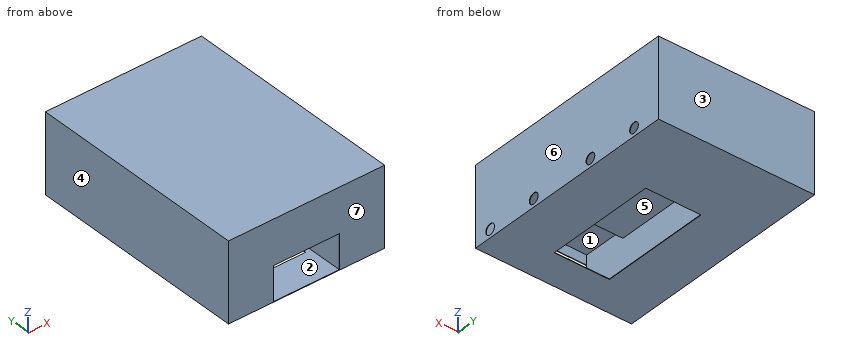
from build123d import *

# Parameters (mm, degrees)
F0_W      = 297
F0_H      = 420
F1_DEPTH  = 150
F3_START  = -1
F2_W      = 295
F2_H      = 418
F3_DEPTH  = 148
F4_W      = 125
F4_H      = 65
F5_DEPTH  = 25
F6_W      = 105
F6_H      = 210
F7_DEPTH  = 25
F9_DEPTH  = 67.5
F11_DEPTH = 295
F12_W     = 83
F12_H     = 1
F13_DEPTH = 148.5
F15_W     = 83
F15_H     = 15.0031849133
F16_DEPTH = 295
F14_W     = 83
F14_H     = 20
F17_DEPTH = 62.5
F18_R     = 10
F19_DEPTH = 7.5


with BuildPart() as f1:
    # F0 (on Top) → F1 (new body)
    with BuildSketch(Plane.XY):
        Rectangle(F0_W, F0_H)
    extrude(amount=F1_DEPTH)

    # F2 (on face) → F3 (cut)
    with BuildSketch(Plane.XY.offset(150).offset(F3_START)):
        Rectangle(F2_W, F2_H)
    extrude(amount=-F3_DEPTH, mode=Mode.SUBTRACT)

    # F4 (on face) → F5 (cut)
    with BuildSketch(Plane.XZ.offset(210)):
        with Locations((0, 33.5)):
            Rectangle(F4_W, F4_H)
    extrude(amount=-F5_DEPTH, mode=Mode.SUBTRACT)

    # F6 (on Top) → F7 (cut)
    with BuildSketch(Plane.XY):
        with Locations((0, -40)):
            Rectangle(F6_W, F6_H)
    extrude(amount=F7_DEPTH, mode=Mode.SUBTRACT)

    # F8 (on face) → F9 (join)
    with BuildSketch(Plane.XY.offset(1)):
        Polygon((-63.5, -209), (-62.5, -209), (-62.5, 65), (61.5036363636, 65), (62.5, -209), (63.5, -209), (62.5, 66), (-63.5, 66), align=None)
    extrude(amount=F9_DEPTH)

    # F10 (on face) → F11 (join, through all)
    with BuildSketch(Plane.YZ.offset(-147.5)):
        Polygon((-126, 68.5), (66, 68.5), (66, 69.5), (-125, 69.5), (-125, 85.5), (-209, 85.5), (-209.0797476204, 84.5031849133), (-126, 84.5031849133), align=None)
    extrude(amount=F11_DEPTH)

    # F12 (on Right) → F13 (join, symmetric)
    with BuildSketch(Plane.YZ):
        with Locations((-167.5, 69)):
            Rectangle(F12_W, F12_H)
    extrude(amount=F13_DEPTH, both=True)

    # F15 (on face) → F16 (join, through all)
    with BuildSketch(Plane.YZ.offset(-147.5)):
        with Locations((-167.5, 77.0015924567)):
            Rectangle(F15_W, F15_H)
    extrude(amount=F16_DEPTH)

    # F14 (on Right) → F17 (cut, symmetric)
    with BuildSketch(Plane.YZ):
        with Locations((-167.5, 74.5)):
            Rectangle(F14_W, F14_H)
    extrude(amount=F17_DEPTH, both=True, mode=Mode.SUBTRACT)

    # F18 (on face) → F19 (cut)
    with BuildSketch(Plane.YZ.offset(148.5)):
        with Locations((-176.1964619943, 15.5)):
            Circle(F18_R)
        with Locations((-76.1964619943, 15.5)):
            Circle(F18_R)
        with Locations((53.8035380057, 15.5)):
            Circle(F18_R)
        with Locations((153.8035380057, 15.5)):
            Circle(F18_R)
    extrude(amount=-F19_DEPTH, mode=Mode.SUBTRACT)


solid = f1.part
Check sheet for the modelled part. Datum: model origin and axes. Units: mm. Face numbers are marked on the shaded views. A direction names the side the tool comes from. Give positions to 0.01 mm unless a question says otherwise; leave off trailing zeros. Loops run counter-clockwise (first coordinate to the right, second up) from the corner with the lowest first, then second, coordinate; pieces in that order, holes last. Notation, with made-up numbers: M 39,-31.5 L 53,-31.5 A24 ccw 53,-18.5 Z; hole C 22.25,-2 d9. An arc over 180 degrees is marked long. Return JSON: item names as keys, results as strings. Group by question number.
1. Cross-section at D-D on z = 94. Record the boundary of the cut face in (x, y).
2. Cross-section at C-C on y = -159.5. Record the boundary of the cut face in (x, z), plus the area to 3 significant figures.
3. Go/stop test with a flat-tipped pin: pin 1 (20.5 mm diameter, centred on x = 23.5, z = 38, fed in from -Y). Record where the tip stops, or that it passes through.
4. Thickness scan on L1, parallel to Z at x = 109, y = -63.5; L2, parallel to Z at x = 57.5, y = -158; L3, parallel to Y at x = 45, z = 81. Record the ranges inside material, lowest first.
5. Mould release check, pull along X, two halves, no side actions. Record for the marked faces 4, 5, 6 and 7: released by +X, released by -X, zero draft, split by the parting line, or undercut.
6. Cross-section at A-A on x = 42. Record the boundary of the cut face in (y, z).
7. Cross-section at B-B on z = 15.5. State how many separate pieces and enclosed holes the cut face has, plus the area to 3 significant figures.
8. Tool access check on the marked faces 1, 2 and 3. Record the directions out of +Z, -Z, +X, -X, +Y, -Y that give a thin tool (end or side, any length) a straight path to the whole face; none if there is none.
Return value:
{
 "1": {"outline": "M -148.5,-210 L 148.5,-210 L 148.5,210 L -148.5,210 Z; hole M -147.5,-209 L 147.5,-209 L 147.5,209 L -147.5,209 Z"},
 "2": {"outline": "M -148.5,0 L 148.5,0 L 148.5,150 L -148.5,150 Z; hole M -147.5,1 L -63.5,1 L -63.5,68.5 L -147.5,68.5 Z; hole M -147.5,85.5 L 147.5,85.5 L 147.5,149 L -147.5,149 Z; hole M -62.5,1 L 62.32,1 L 62.32,64.5 L 62.5,64.5 L 62.5,84.5 L -62.5,84.5 Z; hole M 63.32,1 L 147.5,1 L 147.5,68.5 L 63.32,68.5 Z", "area": "4,040 mm^2"},
 "3": {"pin 1": "y = 65"},
 "4": {"L1": "0 to 1, 68.5 to 69.5, 149 to 150", "L2": "0 to 1, 84.5 to 85.5, 149 to 150", "L3": "-210 to -209, -126 to -125, 209 to 210"},
 "5": {"face 4": "released by -X", "face 5": "undercut", "face 6": "released by +X", "face 7": "zero draft"},
 "6": {"outline": "M -210,0 L -145,0 L -145,1 L -210,1 Z; M -210,66 L -209,66 L -209,84.5 L -126,84.5 L -126,68.5 L 65,68.5 L 65,0 L 210,0 L 210,150 L -210,150 Z; hole M -209,85.5 L -125,85.5 L -125,69.5 L 66,69.5 L 66,1 L 209,1 L 209,149 L -209,149 Z"},
 "7": {"separate pieces": "4", "enclosed holes": "0", "area": "1,900 mm^2"},
 "8": {"face 1": "none", "face 2": "-Y", "face 3": "+Z, -Z, +X, -X, +Y"}
}
